Autodesk Inventor part; units mm, degrees
ref_plane "YZ Plane" through (0, 0, 0) normal (1, 0, 0) x (0, 1, 0)
ref_plane "XZ Plane" through (0, 0, 0) normal (0, 1, 0) x (-1, 0, 0)
ref_plane "XY Plane" through (0, 0, 0) normal (0, 0, 1) x (1, 0, 0)
sketch "スケッチ1" plane through (0, 0, 0) normal (0, 1, 0) x (-1, 0, 0)
  line L0 (0, 16.5925) -> (16.5925, 0)
  line L1 (0, 16.5925) -> (-16.5925, 0)
  line L2 (-16.5925, 0) -> (-16.5925, -12.5795)
  line L3 (-16.5925, -12.5795) -> (16.5925, -12.5795)
  line L4 (16.5925, -12.5795) -> (16.5925, 0)
  line L5 (0, -18.4139) -> (0, 22.427)
  line L6 (23.2296, 0) -> (-23.2296, 0)
  point P0 (0, 0)
  point P1 (0, -12.5795)
  dimension "d0" = 90
extrude "押し出し1" add sketch "スケッチ1" along normal mid plane 20
shell "シェル1" thickness 2.3 removed faces 4 at (-11.0617, 3.3333, 5.5308) at (-16.5925, 3.3333, -8.3863) at (5.5308, 3.3333, 11.0617) at (16.5925, 3.3333, -4.1932)
sketch "スケッチ3" plane through (16.5925, 10, -12.5795) normal (0, 0, -1) x (-1, 0, 0)
  circle A0 centre (16.5925, -10) radius 4
  dimension "d9" = 8
extrude "押し出し3" cut sketch "スケッチ3" against normal through all
sketch "スケッチ4" plane through (0, 10, 0) normal (0, 1, 0) x (1, 0, 0)
  circle A0 centre (0, -2.4504) radius 4
  line L0 (0, -16.5925) -> (16.5925, 0)
  line L1 (-16.5925, 0) -> (0, -16.5925)
  point P0 (0, 0)
  dimension "d12" = 10
  dimension "d13" = 10
  dimension "d14" = 8
extrude "押し出し4" cut sketch "スケッチ4" against normal through all
fillet "フィレット1" radius 8 2 edges at (0, 8.85, 16.5925) (0, -8.85, 16.5925)
properties part number "clip" material "アルミニウム 6061"
Check sheet for the modelled part. Datum: model origin and axes. Units: mm. A direction names the side the tool comes from. Coordinates: 2 decimals unless noted, no trailing zeros. Write each loop counter-clockwise with the first axis right and the second up, starting at its lowest first coordinate (ties: lowest second). Pieces come first, ordered by that corner, then holes. Notation, with made-up numbers: M -17,61 L 11,61 A27 cw 11,94 Z; hole C 67.25,-1 d7. An arc over 180 degrees is marked long. Write item = value, one per line. Start each with the question number.
1. Sectioned sample at C-C (x = 0). Record the cut outline in (y, z).
2. Mould release check, pull along Z, two halves, no side actions. Record for faces 1 (the flat face through (16.592, 0, -12)), 2 (the cylindrical face through (-0.867, 8.866, 6.355)), 3 (the cylindrical face through (0.09, 8.83, 13.28)): pulls with the +Z half, pulls with the -Z half, needs draft (parallel to the pull), parting line crosses it, or undercut.
3. Tool access check on faces 4 (the cylindrical face through (0.09, -8.87, 13.28)), 5 (the flat face through (0, -7.7, -4)). Record the directions out of +Z, -Z, +X, -X, +Y, -Y that give a thin tool (end or side, any length) a straight path to the whole face; none if there is none.
4. Sectioned sample at A-A (y = 0). Record the cut outline in (x, z).
5. Sectioned sample at D-D (x = 13). Record the cut outline in (y, z), then the cut area to 3 significant figures.
6. Thickness scan on probe 1 along Y at (x, z) = (0, -10.85); probe 2 along Y at (x, z) = (-8.5, 0.25); probe 3 along Z at (x, y) = (0, -8.45). Record the ranges inside material, lowest first.
7. Sectioned sample at B-B (z = 11.5). Record the cut outline in (x, y), then the cut area to 3 significant figures.
8. Go/stop test with flat-tipped pins: pin 1 (1.5 mm diameter, centred on x = -3.5, y = -1.5, fed in from -Z); pin 2 (9 mm diameter, centred on x = 0, y = 0, fed in from +Z); pin 3 (3 mm diameter, centred on y = -6, z = 1, fed in from -X). Record where each tip stops, or that it passes through.
The answers:
q1.outline = M -10,-12.58 L -4,-12.58 L -4,-10.28 L -7.7,-10.28 L -7.7,-1.55 L -10,-1.55 Z; M -10,6.45 L -7.7,6.45 L -7.7,13.28 L -10,13.28 Z; M 4,-12.58 L 10,-12.58 L 10,-1.55 L 7.7,-1.55 L 7.7,-10.28 L 4,-10.28 Z; M 7.7,6.45 L 10,6.45 L 10,13.28 L 7.7,13.28 Z
q2.face_1 = needs draft
q2.face_2 = undercut
q2.face_3 = pulls with the +Z half
q3.face_4 = +Z, +Y, -Y
q3.face_5 = +Z, +X, -X
q4.outline = M -16.59,-12.58 L -4,-12.58 L -4,-10.28 L -16.59,-10.28 Z; M 4,-12.58 L 16.59,-12.58 L 16.59,-10.28 L 4,-10.28 Z
q5.outline = M -10,-12.58 L 10,-12.58 L 10,3.59 L 7.7,3.59 L 7.7,-10.28 L -7.7,-10.28 L -7.7,3.59 L -10,3.59 Z
q5.area = 110 mm²
q6.probe_1 = -10 to -4, 4 to 10
q6.probe_2 = -10 to -7.7, 7.7 to 10
q6.probe_3 = -12.58 to -1.55, 6.45 to 13.28
q7.outline = M -5.03,-10 L 5.03,-10 L 5.03,-7.7 L -5.03,-7.7 Z; M -5.03,7.7 L 5.03,7.7 L 5.03,10 L -5.03,10 Z
q7.area = 46.3 mm²
q8.pin_1 = -12.58
q8.pin_2 = -10.28
q8.pin_3 = through
